The model under review builds one solid part; all positions refer to its coordinate system, in mm. A direction names the side the tool comes from. Give positions to 0.01 mm unless a question says otherwise; leave off trailing zeros. Order: outer loops, then holes, each group sorted by start corner. A loop starts at its lowest first (then second) coordinate and runs counter-clockwise, first axis right, second up. Notation, with made-up numbers: (43.25, 74) - (52.25, 74) arc R9 cw to (52.25, 86) - close; hole circle Ø4 at (-27, -25). An arc over 180 degrees is marked (long way). Use CSV: the item, a comma, the result in double quotes. Start each with the question number.
1. Take a section at A-A, the plane x = -31.75. State the section outline as (y, z) points, then the cut area to 3 significant figures.
2. For pin 1 (8 mm diameter, centred on x = -31.75, y = -33.34, fed in from +Z); pin 2 (8 mm diameter, centred on x = 31.5, y = -32, fed in from +Z); pin 3 (1 mm diameter, centred on x = 23.5, y = -11, fed in from +Z), all flat-tipped, find the tip position at first contact; note any pin that passes through.
3. Take a section at D-D, the plane x = -11.5. State the section outline as (y, z) points, then the cut area to 3 significant figures.
4. Take a section at B-B, the plane y = -40. State the section outline as (x, z) points, then the cut area to 3 significant figures.
5. To check wall thickness, follow line 1 (X direction, y = -35, z = -10); line 2 (X direction, y = -35, z = -8.5); line 3 (X direction, y = -7.5, z = -0.5). State the ranges of each line that lie inside material, in increasing order. Write a range as [from, to].
6. Machinability: for faces 1 (the flat face through (1, -2, -18.732)), 2 (the flat face through (34, -13, -15)), 3 (the flat face through (32, -23, 0)), which of the approach directions +Z, -Z, +X, -X, +Y, -Y give a long, thin tool a straight path to every point of the face, cutting with its end or side? Answer none if there is none.
7. Take a section at C-C, the plane z = -6. Count the separate pieces of the cut face and the enclosed holes in it, then the cut area to 3 significant figures.
8. Draft analysis for pull direction X (two halves, no side actions). For faces 4 (the flat face through (-38.1, -22, -12)), 5 (the flat face through (-1, -24, -22.86)), 6 (the cylindrical face through (-29.003, -10.992, -18.985)), state which applies: released by +X, released by -X, zero draft, split by the parting line, or undercut.
```python
from build123d import *

# Parameters (mm, degrees)
F0_W           = 76.2
F0_H           = 50.8
F1_DEPTH       = 44.45
F2_R           = 19.05
F3_DEPTH       = 31.75
F5_DEPTH       = 62.992
F7_D           = 5.5
F7_DEPTH       = 254
F7_CBORE_D     = 9.75
F7_CBORE_DEPTH = 15
F7_TIP         = 1.6523667023
F8_DEPTH       = 2.54
F9_W           = 4.1275
F9_H           = 4.1275
F10_DEPTH      = 86.36


with BuildPart() as f1:
    # F0 (on Front) → F1 (new body)
    with BuildSketch(Plane.XZ):
        Rectangle(F0_W, F0_H)
    extrude(amount=F1_DEPTH)

    # F2 (on face) → F3 (cut)
    with BuildSketch(Plane.XZ.offset(44.45)):
        Circle(F2_R)
    extrude(amount=-F3_DEPTH, mode=Mode.SUBTRACT)

    # F4 (on face) → F5 (cut)
    with BuildSketch(Plane.XZ.offset(44.45)):
        with BuildLine():
            ThreePointArc((1.5e-09, 25.4), (17.9605122427, 17.9605122416), (25.4, 0))
            Line((25.4, 0), (38.1, 0))
            Line((38.1, 0), (38.1, 25.4))
            Line((38.1, 25.4), (1.5e-09, 25.4))
        make_face()
        with BuildLine():
            ThreePointArc((-25.4, 0), (-17.9605122416, 17.9605122427), (1.5e-09, 25.4))
            Line((1.5e-09, 25.4), (-38.1, 25.4))
            Line((-38.1, 25.4), (-38.1, 0))
            Line((-38.1, 0), (-25.4, 0))
        make_face()
    extrude(amount=-F5_DEPTH, mode=Mode.SUBTRACT)

    # F7
    with Locations(Plane.XY):
        with Locations((-31.75, -11.1125), (-31.75, -33.3375), (31.75, -33.3375), (31.75, -11.1125)):
            CounterBoreHole(F7_D / 2, F7_CBORE_D / 2, F7_CBORE_DEPTH, depth=F7_DEPTH)
            with Locations((0, 0, -(F7_DEPTH + F7_TIP / 2))):  # 118° drill point
                Cone(0, F7_D / 2, F7_TIP, mode=Mode.SUBTRACT)

    # F8 (cut): a face of the model
    f8_faces = [f1.faces().sort_by_distance(p)[0] for p in [
        (0, -22.225, -25.4),
    ]]
    extrude(f8_faces, amount=-F8_DEPTH, mode=Mode.SUBTRACT)

    # F9 (on face) → F10 (cut)
    with BuildSketch(Plane.YZ.offset(38.1)):
        with Locations((-2.06375, -20.79625)):
            Rectangle(F9_W, F9_H)
    extrude(amount=-F10_DEPTH, mode=Mode.SUBTRACT)


solid = f1.part
```
Determined:
1,outline,"(-44.45, -22.86) - (-36.09, -22.86) - (-36.09, -15) - (-38.21, -15) - (-38.21, 0) - (-44.45, 0) - close; (-30.59, -22.86) - (-13.86, -22.86) - (-13.86, -15) - (-15.99, -15) - (-15.99, 0) - (-28.46, 0) - (-28.46, -15) - (-30.59, -15) - close; (-8.36, -22.86) - (-4.13, -22.86) - (-4.13, -18.73) - (0, -18.73) - (0, 0) - (-6.24, 0) - (-6.24, -15) - (-8.36, -15) - close"
1,area,"620 mm²"
2,pin 1,"stops at z = -15"
2,pin 2,"stops at z = 0"
2,pin 3,"stops at z = 10.78"
3,outline,"(-44.45, -22.86) - (-4.13, -22.86) - (-4.13, -18.73) - (0, -18.73) - (0, 22.65) - (-44.45, 22.65) - (-44.45, 15.19) - (-12.7, 15.19) - (-12.7, -15.19) - (-44.45, -15.19) - close"
3,area,"1,040 mm²"
4,outline,"(-38.1, -22.86) - (38.1, -22.86) - (38.1, 0) - (25.4, 0) arc R25.4 ccw to (-25.4, 0) - (-38.1, 0) - close; hole circle Ø38.1 at (0, 0)"
4,area,"1,620 mm²"
5,line 1,"x = [-38.1, -36.33], [-27.17, -16.21], [16.21, 27.17], [36.33, 38.1]"
5,line 2,"x = [-38.1, -36.33], [-27.17, -17.05], [17.05, 27.17], [36.33, 38.1]"
5,line 3,"x = [-38.1, -35.02], [-28.48, 28.48], [35.02, 38.1]"
6,face 1,"-Z, +X, -X, +Y"
6,face 2,"+Z"
6,face 3,"+Z, +X, +Y, -Y"
7,separate pieces,"1"
7,enclosed holes,"4"
7,area,"1,940 mm²"
8,face 4,"released by -X"
8,face 5,"zero draft"
8,face 6,"undercut"
